Work out the finished part from the listing and answer in its coordinate system (mm). Face numbers are marked on the shaded views. A direction names the side the tool comes from. Coordinates: 2 decimals unless noted, no trailing zeros. Loops run counter-clockwise (first coordinate to the right, second up) from the corner with the lowest first, then second, coordinate; pieces in that order, holes last. Notation, with made-up numbers: (-5.75, 84.25) - (51.25, 84.25) arc R9 ccw to (51.25, 100.25) - close; hole circle Ø5 at (21, 74). An arc over 180 degrees is marked (long way). Write each question's results on one line, items separated by ' | '. Start each with the question number.
1. Find the intervals of material crossed by line 1 along Z through (x, y) = (0, 4) (3 decimals); line 2 along Z through (x, y) = (1.25, 10.5) (3 decimals); line 3 along Y through (x, z) = (1, -6) (3 decimals), in increasing order. Write a range as [from, to].
2. Determine the mould class of the marked faces 1, 2, 3 and 4 for opening direction Z: released by +Z, released by -Z, zero draft, split by the parting line, or undercut.
3. A cutting plane is placed at A-A on y = 27. Determine the outline of the cut face in (x, z) (3 decimals).
4. Each of these flat-tipped pins is pushed along its axis until it touches: P1, Ø2, axis at x = 0, z = 34.29, coming from the -Y side; P2, Ø4, axis at x = 1, z = -3, coming from the -Y side (3 decimals); P3, Ø4, axis at x = 0, z = -34.29, coming from the +Y side. Where does it stop, or does it pass through?
5. Which of the six approach directions +Z, -Z, +X, -X, +Y, -Y give full straight-line access (tool end or side, diameter ignored) to the marked faces 5 and 6?
6. A cutting plane is placed at C-C on z = 16. Determine the outline of the cut face in (x, y) (3 decimals).
7. A cutting plane is placed at B-B on z = 0. Determine the outline of the cut face in (x, y) (3 decimals), then the cut area to 3 significant figures.
Autodesk Inventor part; units mm, degrees
ref_plane "YZ Plane" through (0, 0, 0) normal (1, 0, 0) x (0, 1, 0)
ref_plane "XZ Plane" through (0, 0, 0) normal (0, 1, 0) x (-1, 0, 0)
ref_plane "XY Plane" through (0, 0, 0) normal (0, 0, 1) x (1, 0, 0)
sketch "Sketch1" plane through (0, 0, 0) normal (0, 1, 0) x (-1, 0, 0)
  line L0 (0, 34.29) -> (0, -34.29) construction
  line L1 (-4.445, 38.735) -> (4.445, 38.735)
  line L2 (4.445, 38.735) -> (4.445, 29.845)
  line L3 (4.445, 29.845) -> (-4.445, 29.845)
  line L4 (-4.445, 29.845) -> (-4.445, 38.735)
  line L5 (-4.445, 38.735) -> (4.445, 29.845) construction
  line L6 (4.445, 38.735) -> (-4.445, 29.845) construction
  line L7 (-4.445, -29.845) -> (4.445, -29.845)
  line L8 (4.445, -29.845) -> (4.445, -38.735)
  line L9 (4.445, -38.735) -> (-4.445, -38.735)
  line L10 (-4.445, -38.735) -> (-4.445, -29.845)
  line L11 (-4.445, -29.845) -> (4.445, -38.735) construction
  line L12 (4.445, -29.845) -> (-4.445, -38.735) construction
  point P0 (0, 0)
  point P1 (0, 0)
  dimension "d0" = 68.58
  dimension "d1" = 8.89
  dimension "d2" = 8.89
  dimension "d3" = 8.89
sketch "Sketch2" plane through (0, 0, 0) normal (1, 0, 0) x (0, 1, 0)
  line L0 (0, 0) -> (63.5, 0) construction
  line L1 (0, 34.29) -> (27.94, 34.29)
  line L2 (0, -34.29) -> (27.94, -34.29)
  line L3 (63.5, 19.05) -> (63.5, -19.05)
  arc A0 (63.5, 19.05) -> (27.94, 34.29) centre (27.94, -14.8167) ccw
  arc A1 (27.94, -34.29) -> (63.5, -19.05) centre (27.94, 14.8167) ccw
  dimension "d4" = 63.5
  dimension "d21" = 38.1
  dimension "d22" = 27.94
  dimension "d23" = 27.94
sweep "Sweep1" add profiles "Sketch1" path "Sketch2" contours L7 L8 L9 L10
sketch "Sketch3" plane through (-4.445, 0, -29.845) normal (0, -1, 0) x (1, 0, 0)
  line L0 (0, 0) -> (0, -8.89)
  circle A0 centre (4.445, -4.445) radius 1.27
  line L1 (0, 68.58) -> (0, 59.69)
  circle A1 centre (4.445, 64.135) radius 1.27
  point P0 (4.445, 29.845)
  dimension "d10" = 2.54
  dimension "d11" = 2.54
  dimension "d12" = 4.445
  dimension "d13" = 34.29
  dimension "d14" = 4.445
  dimension "d15" = 34.29
extrude "Extrusion1" cut sketch "Sketch3" against normal blind 8.89
sketch "Sketch5" plane through (-4.445, 67.945, 20.828) normal (0, 1, 0) x (1, 0, 0)
  circle A0 centre (4.445, 20.828) radius 1.27
  dimension "d24" = 2.54
hole "Hole1" at (0, 67.945, 0) direction (0, -1, 0) diameter 2.54 end through all
properties part number "hpart"
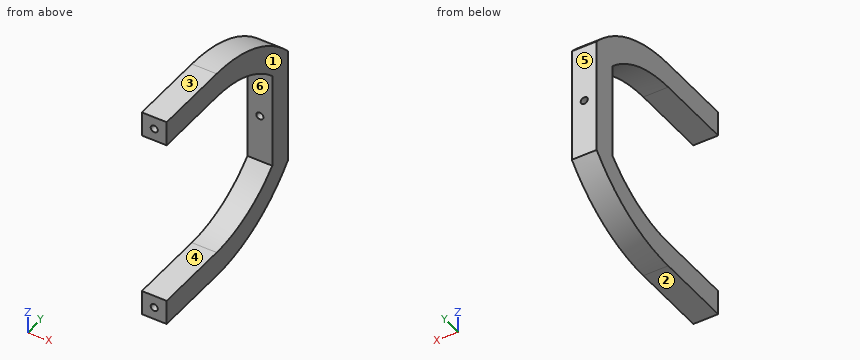
Values:
1) line 1: [-38.735, -35.56], [-33.02, -29.845], [29.845, 33.02], [35.56, 38.735] | line 2: [-38.735, -29.845], [29.845, 38.735] | line 3: [59.055, 67.945]
2) face 1: zero draft | face 2: released by -Z | face 3: released by +Z | face 4: undercut
3) outline: (-4.445, -38.735) - (4.445, -38.735) - (4.445, -29.845) - (-4.445, -29.845) - close; (-4.445, 29.845) - (4.445, 29.845) - (4.445, 38.735) - (-4.445, 38.735) - close
4) P1: y = 8.89 | P2: y = 59.055 | P3: y = 53.41
5) face 5: +Z, -Z, +X, -X, +Y | face 6: +X, -X, -Y
6) outline: (-4.445, 59.055) - (4.445, 59.055) - (4.445, 67.945) - (-4.445, 67.945) - close
7) outline: (-4.445, 59.055) - (-1.27, 59.055) - (-1.27, 67.945) - (-4.445, 67.945) - close; (1.27, 59.055) - (4.445, 59.055) - (4.445, 67.945) - (1.27, 67.945) - close | area: 56.5 mm^2
